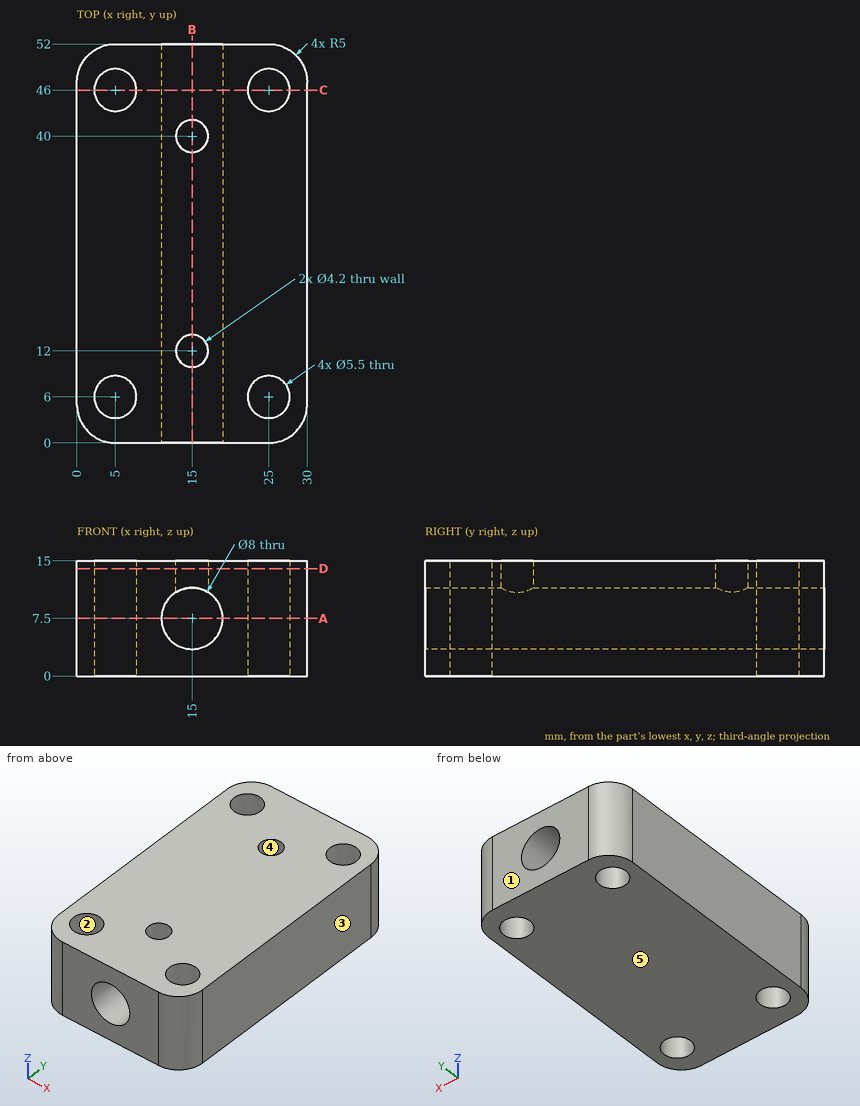
Drawing for the job (mm, zero at the part's lowest x, y, z). A direction names the side the tool comes from. Coordinates: 2 decimals unless noted, no trailing zeros. Order: outer loops, then holes, each group sorted by start corner. A loop starts at its lowest first (then second) coordinate and runs counter-clockwise, first axis right, second up. Notation, with made-up numbers: (-32.5, 38.25) - (23.5, 38.25) arc R18 ccw to (23.5, 47.25) - close; hole circle Ø5 at (55, 41.5). An arc over 180 degrees is marked (long way). Use a Markdown table: item, result. Add a question column.
(1) Which spindle directions (+Z, -Z, +X, -X, +Y, -Y) get a long thin tool onto all of the face, cutting with end or side? Do the marked faces 4 and 5. Say none if no direction does.
(2) Pull direction X, two halves, no side cores. Call the marked faces 1, 2 and 3: +X half, -X half, draft (parallel to the pull), parting line (faces both ways), or undercut.
(3) Drill centre lines: line 1 along Y through (x, z) = (5, 7); line 2 along X through (y, z) = (17.5, 7.75); line 3 along X through (y, z) = (8, 10.5). Where is each one in solid material? Low to high. Write a range as [from, to].
(4) Saw through at C-C (y = 46). Give the cut face in (x, z).
(5) Saw through at B-B (x = 15). Give the cut face in (y, z).
(6) Saw through at A-A (z = 7.5). Give the cut face in (x, y), then the cut area to 3 significant figures.
(7) Saw through at D-D (z = 14). Give the cut face in (x, y).
Solved:
| question | item | result |
|---|---|---|
| 1 | face 4 | +Z |
| 1 | face 5 | -Z, +X, -X, +Y, -Y |
| 2 | face 1 | draft |
| 2 | face 2 | undercut |
| 2 | face 3 | +X half |
| 3 | line 1 | y = [0, 3.25], [8.75, 43.25], [48.75, 52] |
| 3 | line 2 | x = [0, 11.01], [18.99, 30] |
| 3 | line 3 | x = [0, 3.11], [6.89, 12.35], [17.65, 23.11], [26.89, 30] |
| 4 | outline | (0, 0) - (2.25, 0) - (2.25, 15) - (0, 15) - close; (7.75, 0) - (22.25, 0) - (22.25, 15) - (7.75, 15) - close; (27.75, 0) - (30, 0) - (30, 15) - (27.75, 15) - close; hole circle Ø8 at (15, 7.5) |
| 5 | outline | (0, 0) - (52, 0) - (52, 3.5) - (0, 3.5) - close; (0, 11.5) - (9.9, 11.5) - (9.9, 15) - (0, 15) - close; (14.1, 11.5) - (37.9, 11.5) - (37.9, 15) - (14.1, 15) - close; (42.1, 11.5) - (52, 11.5) - (52, 15) - (42.1, 15) - close |
| 6 | outline | (0, 5) arc R5 ccw to (5, 0) - (11, 0) - (11, 52) - (5, 52) arc R5 ccw to (0, 47) - close; (19, 0) - (25, 0) arc R5 ccw to (30, 5) - (30, 47) arc R5 ccw to (25, 52) - (19, 52) - close; hole circle Ø5.5 at (5, 6); hole circle Ø5.5 at (5, 46); hole circle Ø5.5 at (25, 6); hole circle Ø5.5 at (25, 46) |
| 6 | area | 1,030 mm² |
| 7 | outline | (0, 5) arc R5 ccw to (5, 0) - (25, 0) arc R5 ccw to (30, 5) - (30, 47) arc R5 ccw to (25, 52) - (5, 52) arc R5 ccw to (0, 47) - close; hole circle Ø5.5 at (5, 6); hole circle Ø5.5 at (5, 46); hole circle Ø4.2 at (15, 12); hole circle Ø4.2 at (15, 40); hole circle Ø5.5 at (25, 6); hole circle Ø5.5 at (25, 46) |
